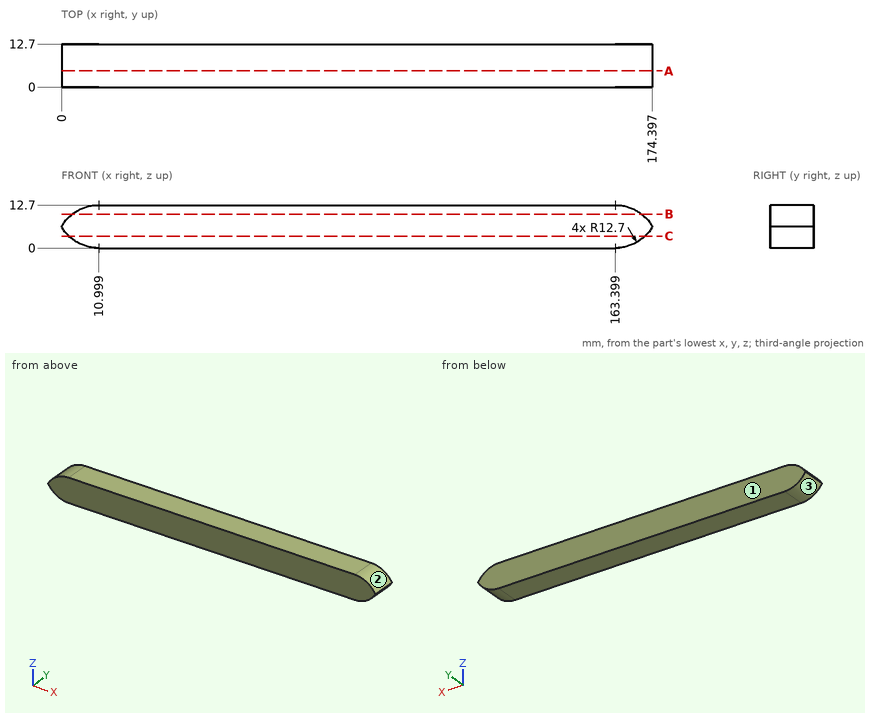
Could you check a few things on this drawing? It's one solid part, dimensions in mm from its lowest x, y, z. Give positions to 0.01 mm unless a question says otherwise; leave off trailing zeros. Write each loop counter-clockwise with the first axis right and the second up, starting at its lowest first coordinate (ties: lowest second). Pieces come first, ordered by that corner, then holes. Notation, with made-up numbers: (-15.75, 35.25) -> (24.25, 35.25) arc R31 ccw to (24.25, 72.25) -> close; hole circle Ø3 at (57.5, -12). An arc over 180 degrees is marked (long way). Answer as CSV lines item,"result". Start each with the question number.
(1) Please list where these lines run through material, in increasing order: line 1 (X direction, y = 10.25, z = 6.5); line 2 (X direction, y = 1.5, z = 4.5) (1 decimal).
(2) If we section it at B-B, the plane z = 10: Write out the boundary of the cut face in (x, y), and give its area (3 significant figures).
(3) I'm going to push flat-ended pins straight in: pin 1 Ø1 at (y, z) = (3, 8) entering from -X; pin 2 Ø2 at (y, z) = (5, 8) entering from -X; pin 3 Ø5 at (y, z) = (8, 7.5) entering from +X. Where does each tip first touch, or does it pass through?
(4) If we mould it in two halves opening along X, with no side actions, what happens to the marked faces 1, 2 and 3? For each: +X half, -X half, draft (parallel to the pull), parting line (faces both ways), or undercut.
(5) If we section it at A-A, the plane y = 4.75: Write out the boundary of the cut face in (x, z).
(6) If we section it at C-C, the plane z = 3.5: Write out the boundary of the cut face in (x, y).
Answer list:
1,line 1,"0.09 to 174.31"
1,line 2,"1.3 to 173.1"
2,outline,"(3.17, 0) -> (171.23, 0) -> (171.23, 12.7) -> (3.17, 12.7) -> close"
2,area,"2,130 mm^2"
3,pin 1,"x = 0.75"
3,pin 2,"x = 0.4"
3,pin 3,"x = 174.4"
4,face 1,"draft"
4,face 2,"+X half"
4,face 3,"-X half"
5,outline,"(0, 6.35) arc R12.7 ccw to (11, 0) -> (163.4, 0) arc R12.7 ccw to (174.4, 6.35) arc R12.7 ccw to (163.4, 12.7) -> (11, 12.7) arc R12.7 ccw to start"
6,outline,"(2.24, 0) -> (172.15, 0) -> (172.15, 12.7) -> (2.24, 12.7) -> close"
